Can you work these out from the model? Positions are in its coordinate system, mm. Coordinates: 2 decimals unless noted, no trailing zeros. Order: outer loops, then holes, each group sorted by start corner. A loop starts at its lowest first (then second) coordinate and runs counter-clockwise, first axis right, second up. Notation, with made-up numbers: (20, 43) -> (52, 43) arc R37 ccw to (52, 82) -> close; hole circle Ø9 at (38.25, -8.5). An arc over 180 degrees is marked (long way). Return JSON: item names as keys, results as strings. Group by question number.
1) If we section it at A-A, the plane z = 528: Please give me the cut outline in (x, y).
2) Thinking about a two-plate mould opening in X: for faces 1 (the flat face through (1167, -9, 560)), 2 (the flat face through (776, -19, 492)), 3 (the flat face through (777, -9, 563)), 4 (the flat face through (395, -9, 560)), which applies, +X half, -X half, draft (parallel to the pull), parting line (faces both ways), or undercut?
3) If we section it at D-D, the plane z = 480.5: Please give me the cut outline in (x, y), then the cut area to 3 significant figures.
4) For pin 1 (10 mm diameter, centred on x = 1040.5, y = -22.5, fed in from -Z); pin 2 (8 mm diameter, centred on y = -25.5, z = 560.5, fed in from -X); pin 3 (6 mm diameter, centred on x = 544, z = 600, fed in from -Y), each with a flat end and sliding along its axis, tell me the tip position at first contact or that it passes through.
5) If we section it at B-B, the plane x = 794: Please give me the cut outline in (y, z), then the cut area to 3 significant figures.
6) If we section it at C-C, the plane z = 569: State how many separate pieces and enclosed holes the cut face has, then the cut area to 3 significant figures.
7) If I drill on probe 1 along Z at (x, y) = (477, -10); probe 2 along X at (y, z) = (-18.5, 572); probe 3 along Y at (x, z) = (562.5, 590), over which ranges is the centre line in solid material (lowest first)? Write a range as from..to.
from build123d import *

# Parameters (mm, degrees)
CLONE2D004_W    = 772
CLONE2D004_H    = 216
PAD012_DEPTH    = 19
SKETCH029_W     = 622
SKETCH029_H     = 116
POCKET012_DEPTH = 10


with BuildPart() as part:
    # Clone2D004 → Pad012 (new body)
    with BuildSketch(Plane.XZ):
        with Locations((386, 108)):
            Rectangle(CLONE2D004_W, CLONE2D004_H)
    extrude(amount=PAD012_DEPTH)

    # Sketch029 (on Face6 of Pad012) → Pocket012 (cut)
    with BuildSketch(Plane.XZ.offset(19)):
        with Locations((386, 108)):
            Rectangle(SKETCH029_W, SKETCH029_H)
    extrude(amount=-POCKET012_DEPTH, mode=Mode.SUBTRACT)

    # Clone2D005 → Revolution002 (revolve)
    with BuildSketch(Plane(origin=(175, -9, 107.5), x_dir=(1, 0, 0), z_dir=(0, 0, 1))):
        with BuildLine():
            Line((0, 0), (0, -20))
            add(Edge.make_bspline(
                [(0, -20), (-18, -20), (-18, -9.133286), (-4.506424, -9.133286), (-7.5, 0)],
                knots=[0, 0, 0, 0, 0.5, 1, 1, 1, 1], degree=3, weights=[7, 6.116989, 5.810816, 6.060123, 5.999522]))
            Line((-7.5, 0), (0, 0))
        make_face()
    revolve(axis=Axis((175, -9, 107.5), (0, 1, 0)))

    # Clone2D006 → Revolution003 (revolve)
    with BuildSketch(Plane(origin=(574, -9, 107.5), x_dir=(1, 0, 0), z_dir=(0, 0, 1))):
        with BuildLine():
            Line((0, 0), (0, -20))
            add(Edge.make_bspline(
                [(0, -20), (-18, -20), (-18, -9.133286), (-4.506424, -9.133286), (-7.5, 0)],
                knots=[0, 0, 0, 0, 0.5, 1, 1, 1, 1], degree=3, weights=[7, 6.116989, 5.810816, 6.060123, 5.999522]))
            Line((-7.5, 0), (0, 0))
        make_face()
    revolve(axis=Axis((574, -9, 107.5), (0, 1, 0)))


with BuildPart() as part_1:
    # Body012 placement: moved
    add(part.part.moved(Location((394, 0, 10))))


with BuildPart() as part_2:
    # Clone placement: moved
    add(part_1.part.moved(Location((-393, 0, -10))))


with BuildPart() as part_3:
    # Body013 placement: moved
    add(part_2.part.moved(Location((394, 0, 454))))


solid = part_3.part
Result sheet:
{
 "1": {"outline": "(395, -19) -> (470, -19) -> (470, -9) -> (1092, -9) -> (1092, -19) -> (1167, -19) -> (1167, 0) -> (395, 0) -> close"},
 "2": {"face 1": "+X half", "face 2": "draft", "face 3": "undercut", "face 4": "-X half"},
 "3": {"outline": "(395, -19) -> (1167, -19) -> (1167, 0) -> (395, 0) -> close", "area": "14,700 mm2"},
 "4": {"pin 1": "stops at z = 454", "pin 2": "stops at x = 553.73", "pin 3": "stops at y = -9"},
 "5": {"outline": "(-19, 454) -> (0, 454) -> (0, 670) -> (-19, 670) -> (-19, 620) -> (-9, 620) -> (-9, 504) -> (-19, 504) -> close", "area": "2,940 mm2"},
 "6": {"separate pieces": "3", "enclosed holes": "0", "area": "8,970 mm2"},
 "7": {"probe 1": "z = 454..504, 620..670", "probe 2": "x = 395..470, 1092..1167", "probe 3": "y = -9..0"}
}
